Source: CAD feature listing. Evaluate the final solid. Frame: model axes, mm. A direction names the side the tool comes from. Coordinates: 2 decimals unless noted, no trailing zeros. Loops run counter-clockwise (first coordinate to the right, second up) from the corner with the lowest first, then second, coordinate; pieces in that order, holes last.
Item 1: Line query: probe 1 along Z at (x, y) = (-69, -0.25); probe 2 along Z at (x, y) = (135.5, -1.75); probe 3 along X at (y, z) = (3, -7.5). Output: solid intervals per line, ascending.
Item 2: Reachability of faces 4 (the cylindrical face through (145, 4, 0)), 5 (the flat face through (-135, 0, -4)), 6 (the conical face through (125.313, 5.067, 1.596)) from +Z, -Z, +X, -X, +Y, -Y: full face, straight path, thin tool, end or side. Return the list, or none.
Item 3: Section query A-A, the plane z = 0. Return the cut outline in (x, y), then the cut area to 3 significant figures.
Item 4: Pin query (flat end, axial travel): pin 1 Ø1.5 at (x, z) = (-60, 2) entering from +Y; pin 2 Ø2 at (x, z) = (-80, -1.5) entering from +Y; pin 3 Ø1.5 at (y, z) = (-7, -5.5) entering from -X. Return the tip coordinate at first contact, or that it passes through.
Item 5: Section query B-B, the plane x = 67.5. Return the cut outline in (y, z).
Item 6: Pull-direction query (X, two-part tool) for faces 1 (the flat face through (135, 0, -4)), 2 (the cylindrical face through (132.54, -2.17, -9.76)), 3 (the conical face through (-125.24, 5, 1.57)); classes: +X half, -X half, draft (parallel to the pull), parting line (faces both ways), or undercut.
```python
from build123d import *

# Parameters (mm, degrees)
SKETCH3_R               = 4
BOSS_EXTRUDE3_DEPTH     = 5
SKETCH2_W               = 25
SKETCH2_H               = 0.75
SKETCH2_W_2             = 20
CUT_EXTRUDE1_DEPTH      = 11
CUT_EXTRUDE1_DEPTH_BACK = 11


with BuildPart() as part:
    # Sketch1 → Revolve3 (revolve)
    with BuildSketch(Plane.XY):
        Polygon((-125, 5), (125, 5), (130, 10), (135, 10), (135, 4), (155, 4), (155, 0), (-155, 0), (-155, 4), (-135, 4), (-135, 10), (-130, 10), align=None)
    revolve(axis=Axis((-25.367414289, 0, 0), (1, 0, 0)))

    # Sketch3 → Boss-Extrude3 (add)
    with BuildSketch(Plane.ZY.offset(155)):
        Circle(SKETCH3_R)
    extrude(amount=BOSS_EXTRUDE3_DEPTH)

    # Sketch2 → Cut-Extrude1 (cut, two sides)
    with BuildSketch(Plane(origin=(0, 0, 0), x_dir=(1, 0, 0), z_dir=(0, 1, 0))) as cut_extrude1_sk:
        with Locations((-147.5, 3.625)):
            Rectangle(SKETCH2_W, SKETCH2_H)
        with Locations((145, -3.625)):
            Rectangle(SKETCH2_W_2, SKETCH2_H)
        with Locations((145, 3.625)):
            Rectangle(SKETCH2_W_2, SKETCH2_H)
        with Locations((-147.5, -3.625)):
            Rectangle(SKETCH2_W, SKETCH2_H)
    extrude(amount=CUT_EXTRUDE1_DEPTH, mode=Mode.SUBTRACT)
    extrude(cut_extrude1_sk.sketch, amount=-CUT_EXTRUDE1_DEPTH_BACK, mode=Mode.SUBTRACT)


solid = part.part
```
Verdict:
1. probe 1: z = -4.99 to 4.99
1. probe 2: z = -3.25 to 3.25
1. probe 3: x = -135 to -128.08, 128.08 to 135
2. face 4: +X, +Y
2. face 5: -X
2. face 6: none
3. outline: (-160, -4) - (-135, -4) - (-135, -10) - (-130, -10) - (-125, -5) - (125, -5) - (130, -10) - (135, -10) - (135, -4) - (155, -4) - (155, 4) - (135, 4) - (135, 10) - (130, 10) - (125, 5) - (-125, 5) - (-130, 10) - (-135, 10) - (-135, 4) - (-160, 4) - close
3. area: 3,210 mm2
4. pin 1: stops at y = 4.84
4. pin 2: stops at y = 4.97
4. pin 3: stops at x = -135
5. outline: circle Ø10 at (0, 0)
6. face 1: +X half
6. face 2: draft
6. face 3: undercut
